```python
from build123d import *

# Parameters (mm, degrees)
SKETCH_W        = 110
SKETCH_H        = 64
SKETCH_R        = 1.75
PAD_DEPTH       = 3
CHAMFER_SIZE    = 1.5
FILLET_R        = 2
SKETCH001_W     = 83
SKETCH001_H     = 3
PAD001_DEPTH    = 86
FILLET001_R     = 1
SKETCH002_R     = 2
POCKET_DEPTH    = 5
POCKET001_DEPTH = 5
FILLET002_R     = 1
SKETCH004_W     = 35
SKETCH004_H     = 53
POCKET002_DEPTH = 5
FILLET003_R     = 1
SKETCH005_W     = 2.8
SKETCH005_H     = 87.98
PAD002_DEPTH    = 3.16
FILLET004_R     = 1


with BuildPart() as part:
    # Sketch → Pad (new body)
    with BuildSketch(Plane.XY):
        Rectangle(SKETCH_W, SKETCH_H)
        with Locations((-45, 0)):
            Circle(SKETCH_R, mode=Mode.SUBTRACT)
        with Locations((45, 0)):
            Circle(SKETCH_R, mode=Mode.SUBTRACT)
    extrude(amount=PAD_DEPTH)

    # Chamfer
    chamfer_edges = [part.edges().sort_by_distance(p)[0] for p in [
        (43.25, 0, 3),
        (-46.75, 0, 3),
    ]]
    chamfer(chamfer_edges, length=CHAMFER_SIZE)

    # Fillet
    fillet_edges = [part.edges().sort_by_distance(p)[0] for p in [
        (-55, 32, 1.5),
        (0, 32, 3),
        (55, 32, 1.5),
        (55, 0, 3),
        (0, -32, 3),
        (-55, 0, 3),
        (-55, -32, 1.5),
        (55, -32, 1.5),
    ]]
    fillet(fillet_edges, radius=FILLET_R)

    # Sketch001 (on Face22 of Fillet) → Pad001 (join)
    with BuildSketch(Plane.XY.offset(3)):
        with Locations((0, 27.34)):
            Rectangle(SKETCH001_W, SKETCH001_H)
    extrude(amount=PAD001_DEPTH)

    # Fillet001
    fillet001_edges = [part.edges().sort_by_distance(p)[0] for p in [
        (-41.5, 25.84, 46),
        (-41.5, 28.84, 46),
        (-41.5, 27.34, 89),
        (0, 28.84, 89),
        (0, 25.84, 89),
        (41.5, 25.84, 46),
        (41.5, 28.84, 46),
        (41.5, 27.34, 89),
    ]]
    fillet(fillet001_edges, radius=FILLET001_R)

    # Sketch002 (on Face6 of Fillet001) → Pocket (cut)
    with BuildSketch(Plane(origin=(0, 28.84, 0), x_dir=(-1, 0, 0), z_dir=(0, 1, 0))):
        with Locations((-29.5, 59)):
            Circle(SKETCH002_R)
        with Locations((29.5, 59)):
            Circle(SKETCH002_R)
    extrude(amount=-POCKET_DEPTH, mode=Mode.SUBTRACT)

    # Sketch003 (on Face5 of Pocket) → Pocket001 (cut)
    with BuildSketch(Plane.XZ.offset(-25.84)):
        with BuildLine():
            Line((7, 24.84), (7, 3))
            Line((7, 3), (-7, 3))
            Line((-7, 3), (-7, 24.84))
            ThreePointArc((7, 24.84), (0, 31.920457), (-7, 24.84))
        make_face()
    extrude(amount=-POCKET001_DEPTH, mode=Mode.SUBTRACT)

    # Fillet002
    fillet002_edges = [part.edges().sort_by_distance(p)[0] for p in [
        (0, 25.84, 31.920457),
        (-7, 25.84, 13.92),
        (7, 25.84, 13.92),
        (-7, 28.84, 13.92),
        (0, 28.84, 31.920457),
        (7, 28.84, 13.92),
    ]]
    fillet(fillet002_edges, radius=FILLET002_R)

    # Sketch004 (on Face7 of Fillet002) → Pocket002 (cut)
    with BuildSketch(Plane(origin=(0, 28.84, 0), x_dir=(-1, 0, 0), z_dir=(0, 1, 0))):
        with Locations((0, 66.71)):
            Rectangle(SKETCH004_W, SKETCH004_H)
    extrude(amount=-POCKET002_DEPTH, mode=Mode.SUBTRACT)

    # Fillet003
    fillet003_edges = [part.edges().sort_by_distance(p)[0] for p in [
        (0, 28.84, 40.21),
        (0, 25.84, 40.21),
        (-17.5, 27.34, 40.21),
        (-17.5, 28.84, 64.105),
        (-17.5, 25.84, 64.105),
        (17.5, 28.84, 64.105),
        (17.5, 28.547107, 88.707107),
        (17.5, 27.34, 89),
        (-17.5, 28.547107, 88.707107),
        (-17.5, 27.34, 89),
        (-17.5, 26.132893, 88.707107),
        (17.5, 27.34, 40.21),
        (17.5, 25.84, 64.105),
        (17.5, 26.132893, 88.707107),
    ]]
    fillet(fillet003_edges, radius=FILLET003_R)

    # Sketch005 (on Face25 of Fillet003) → Pad002 (join)
    with BuildSketch(Plane(origin=(0, 28.84, 0), x_dir=(-1, 0, 0), z_dir=(0, 1, 0))):
        with Locations((-39.1, 43.99)):
            Rectangle(SKETCH005_W, SKETCH005_H)
        with Locations((-19.91, 43.99)):
            Rectangle(SKETCH005_W, SKETCH005_H)
        with Locations((19.91, 43.99)):
            Rectangle(SKETCH005_W, SKETCH005_H)
        with Locations((39.09, 43.99)):
            Rectangle(SKETCH005_W, SKETCH005_H)
    extrude(amount=PAD002_DEPTH)

    # Fillet004
    fillet004_edges = [part.edges().sort_by_distance(p)[0] for p in [
        (40.5, 30.42, 87.98),
        (39.1, 32, 87.98),
        (37.7, 30.42, 87.98),
        (21.31, 30.42, 87.98),
        (19.91, 32, 87.98),
        (18.51, 30.42, 87.98),
        (-18.51, 30.42, 87.98),
        (-19.91, 32, 87.98),
        (-21.31, 30.42, 87.98),
        (-37.69, 30.42, 87.98),
        (-39.09, 32, 87.98),
        (-40.49, 30.42, 87.98),
    ]]
    fillet(fillet004_edges, radius=FILLET004_R)


solid = part.part
```
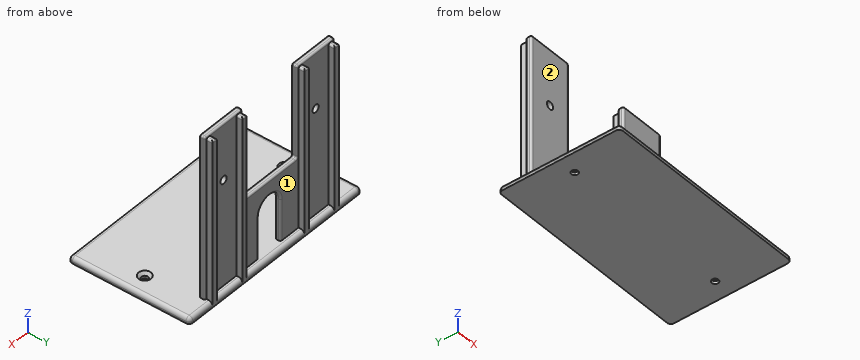
For this review, take the finished solid that the model builds, in its own axes (mm). Face numbers are marked on the shaded views. Round coordinates to 2 decimals unless told otherwise and drop trailing zeros. Write each loop counter-clockwise with the first axis right and the second up, starting at its lowest first coordinate (ties: lowest second). Pieces come first, ordered by that corner, then holes. Notation, with made-up numbers: (16, 23.5) -> (35, 23.5) arc R20 cw to (35, 44.5) -> close; hole circle Ø1 at (-37.5, -37). An arc over 180 degrees is marked (long way). Use one line per item in the form item = value.
1) Take a section at D-D, the plane y = -24.5. Write out the cut boundary in (x, z).
Found:
outline = (-55, 0) -> (55, 0) -> (55, 1) arc R2 ccw to (53, 3) -> (-53, 3) arc R2 ccw to (-55, 1) -> close
2) To check wall thickness, follow L1, parallel to Y at x = 45, z = 0.5; L2, parallel to Z at x = 23.5, y = 8; L3, parallel to Y at x = -24, z = 21. State the ranges of each line that lie inside material, in increasing order. Write a range as from..to.
Found:
L1 = -32..-1.75, 1.75..32
L2 = 0..3
L3 = 25.84..28.84
3) Mouldability with a two-part tool opening along X and no side actions: class the marked faces 1 and 2 as +X half, -X half, draft (parallel to the pull), parting line (faces both ways), or undercut.
Found:
face_1 = undercut
face_2 = draft
4) Clearance check with flat-ended pins moving along their axes: pin 1 (0.8 mm diameter, centred on y = 27.5, z = 45, fed in from +X); pin 2 (6 mm diameter, centred on x = 22.5, z = 23, fed in from -Y); pin 3 (2.5 mm diameter, centred on y = 31, z = 29, fed in from +X). State where each tip first meets the part, or that it passes through.
Found:
pin_1 = 41.5
pin_2 = 25.84
pin_3 = 40.5
5) Take a section at B-B, the plane x = 0. Write out the cut boundary in (y, z), and give its area (3 significant figures).
Found:
outline = (-32, 0) -> (32, 0) -> (32, 1) arc R2 ccw to (30, 3) -> (-30, 3) arc R2 ccw to (-32, 1) -> close; (25.84, 32.92) arc R1 ccw to (26.84, 31.92) -> (27.84, 31.92) arc R1 ccw to (28.84, 32.92) -> (28.84, 39.21) arc R1 ccw to (27.84, 40.21) -> (26.84, 40.21) arc R1 ccw to (25.84, 39.21) -> close
area = 214 mm2
